Here's how the part is built. I have some questions about the finished solid (model axes, mm). A direction names the side the tool comes from. Give positions to 0.01 mm unless a question says otherwise; leave off trailing zeros. Write each loop counter-clockwise with the first axis right and the second up, starting at its lowest first coordinate (ties: lowest second). Pieces come first, ordered by that corner, then holes. Notation, with made-up numbers: (58.5, 16) -> (67.5, 16) arc R14 ccw to (67.5, 29) -> close; hole circle Ø10 at (9.5, -37.75). An arc over 180 degrees is marked (long way). Use one line per item in the form item = value.
```python
from build123d import *

# Parameters (mm, degrees)
SKETCH004_R     = 4.5
PAD003_DEPTH    = 3
SKETCH005_R     = 15
PAD004_DEPTH    = 2
SKETCH006_R     = 15
SKETCH006_R_2   = 13
PAD005_DEPTH    = 3
SKETCH007_R     = 5
POCKET001_DEPTH = 1
FILLET001_R     = 0.5
CHAMFER001_SIZE = 1


with BuildPart() as part:
    # Sketch004 → Pad003 (new body)
    with BuildSketch(Plane.XY):
        Circle(SKETCH004_R)
        with BuildLine():
            ThreePointArc((-2.078461, 2.3), (0, -3.1), (2.078461, 2.3))
            Line((-2.078461, 2.3), (2.078461, 2.3))
        make_face(mode=Mode.SUBTRACT)
    extrude(amount=PAD003_DEPTH)

    # Sketch005 (on Face5 of Pad003) → Pad004 (join)
    with BuildSketch(Plane.XY.offset(3)):
        Circle(SKETCH005_R)
    extrude(amount=PAD004_DEPTH)

    # Sketch006 (on Face2 of Pad004) → Pad005 (join)
    with BuildSketch(Plane(origin=(0, 0, 3), x_dir=(1, 0, 0), z_dir=(0, 0, -1))):
        Circle(SKETCH006_R)
        Circle(SKETCH006_R_2, mode=Mode.SUBTRACT)
    extrude(amount=PAD005_DEPTH)

    # Sketch007 (on Face3 of Pad005) → Pocket001 (cut)
    with BuildSketch(Plane.XY.offset(5)):
        with Locations((5.303301, 5.303301)):
            Circle(SKETCH007_R)
    extrude(amount=-POCKET001_DEPTH, mode=Mode.SUBTRACT)

    # Fillet001
    fillet001_edges = [part.edges().sort_by_distance(p)[0] for p in [
        (0.303301, 5.303301, 5),
    ]]
    fillet(fillet001_edges, radius=FILLET001_R)

    # Chamfer001
    chamfer001_edges = [part.edges().sort_by_distance(p)[0] for p in [
        (-15, 0, 5),
    ]]
    chamfer(chamfer001_edges, length=CHAMFER001_SIZE)


with BuildPart() as part_1:
    # Body001 placement: moved
    add(part.part.moved(Location((28.4, 0, 0))))


solid = part_1.part
```
Q1. I want a section at B-B, the plane z = 3.45. Write out the boundary of the cut face in (x, y).
Result set:
outline = circle Ø30 at (28.4, 0)
Q2. Will these pins go through, and if not, where does the flat tip stop? pin 1 Ø2 at (x, y) = (26.5, 6.5) entering from -Z; pin 2 Ø1.5 at (x, y) = (36.5, 6.5) entering from +Z; pin 3 Ø2 at (y, z) = (-11, 0.5) entering from -X.
Result set:
pin_1 = 3
pin_2 = 4
pin_3 = 17.22
Q3. Which directions (+Z, -Z, +X, -X, +Y, -Y) give clear straight access to the entire face, cutting with the end or side of a thin tool? Please do faces 1 (the face through (40.4, 5, 1.5)), 2 (the face through (34, 5, 4)), 3 (the face through (17, -7, 0)).
Result set:
face_1 = -Z
face_2 = +Z
face_3 = -Z, +X, -X, +Y, -Y
Q4. If I drill on line 1 along Y through (x, z) = (28.5, 0.85); line 2 along Z through (x, y) = (33.75, 2.5); line 3 along Z through (x, y) = (19.5, -0.25), over which ranges is the centre line in solid material (lowest first)? Write a range as from..to.
Result set:
line_1 = -15..-13, -4.5..-3.1, 2.3..4.5, 13..15
line_2 = 3..4
line_3 = 3..5
Q5. I want a section at A-A, the plane z = 1.4. Write out the boundary of the cut face in (x, y).
Result set:
outline = circle Ø30 at (28.4, 0); circle Ø9 at (28.4, 0); hole circle Ø26 at (28.4, 0); hole (26.32, 2.3) arc R3.1 ccw (long way) to (30.48, 2.3) -> close
